from build123d import *

# Parameters (mm, degrees)
F1_R          = 28.006963647
F2_DEPTH      = 100
F0_R          = 228.6
F3_DEPTH      = 50
F4_R          = 7.5
F5_DEPTH      = 28.006963647
F5_DEPTH_BACK = 28.006963647


with BuildPart() as f2:
    # F1 (on Front) → F2 (new body)
    with BuildSketch(Plane.XZ):
        Circle(F1_R)
    extrude(amount=F2_DEPTH)

    # F0 (on Front) → F3 (join)
    with BuildSketch(Plane.XZ):
        Circle(F0_R)
    extrude(amount=-F3_DEPTH)

    # F4 (on Top) → F5 (cut, two sides)
    with BuildSketch(Plane.XY) as f5_sk:
        with Locations((0, -45)):
            Circle(F4_R)
    extrude(amount=-F5_DEPTH, mode=Mode.SUBTRACT)
    extrude(f5_sk.sketch, amount=F5_DEPTH_BACK, mode=Mode.SUBTRACT)


solid = f2.part
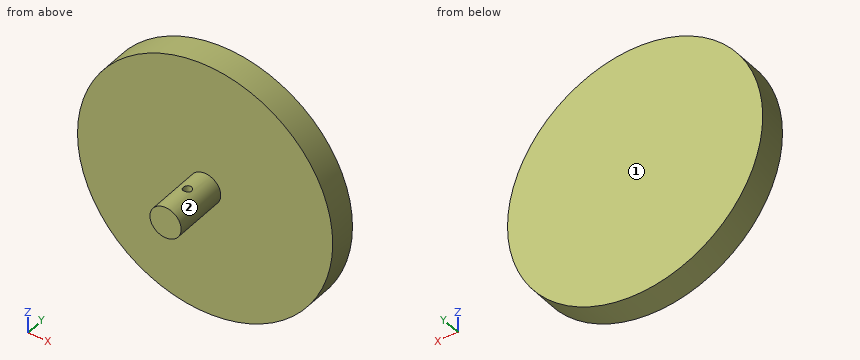
Geometry: final body of the model. Coordinates: model frame, mm. Face numbers are marked on the shaded views. A direction names the side the tool comes from. Round coordinates to 2 decimals unless told otherwise and drop trailing zeros. Loops run counter-clockwise (first coordinate to the right, second up) from the corner with the lowest first, then second, coordinate; pieces in that order, holes last. Notation, with made-up numbers: M 1,-22.5 L 13,-22.5 A25 cw 13,10.5 Z; hole C 5.5,13 d11. An arc over 180 degrees is marked long. Put each result on its own line as item: value. Start each with the question number.
(1) Section query A-A (z = 0). Return loops of the section in (x, y).
(2) Section query B-B (x = 0). Return loops of the section in (y, z).
(3) Section query D-D (y = -18). Return loops of the section in (x, z), then the cut area to 3 significant figures.
(4) Material intervals for line 1 along Y through (x, z) = (0, 0); line 2 along Y through (x, z) = (-159.5, 16); line 3 along X through (y, z) = (-45, 3), sorted ascending. Write a range as [from, to].
(5) Set-up query: the marked faces 1 and 2. Return all of +Z, -Z, +X, -X, +Y, -Y with unobstructed straight access to the full face (end or side cutting, diameter ignored); none if empty.
(6) Section query C-C (y = -45). Return loops of the section in (x, z).
(7) Contact query for flat-ended pins moving along their axis: pin 1 Ø10 at (y, z) = (-38, -16.5) entering from -X; pin 2 Ø24 at (x, y) = (0, -45) entering from +Z; pin 3 Ø5 at (x, y) = (-15.5, -67.5) entering from +Z; pin 4 Ø12 at (x, y) = (136.5, -10) entering from -Z. Output: stop coordinate, or through.
Findings below:
1. outline: M -228.6,0 L -28.01,0 L -28.01,-100 L 28.01,-100 L 28.01,0 L 228.6,0 L 228.6,50 L -228.6,50 Z; hole C 0,-45 d15
2. outline: M -100,-28.01 L -52.5,-28.01 L -52.5,28.01 L -100,28.01 Z; M -37.5,-28.01 L 0,-28.01 L 0,-228.6 L 50,-228.6 L 50,228.6 L 0,228.6 L 0,28.01 L -37.5,28.01 Z
3. outline: C 0,0 d56.01
3. area: 2,460 mm2
4. line 1: y = [-100, -52.5], [-37.5, 50]
4. line 2: y = [0, 50]
4. line 3: x = [-27.85, -7.5], [7.5, 27.85]
5. face 1: +Z, -Z, +X, -X, +Y
5. face 2: -Y
6. outline: M -7.5,-26.98 L -7.5,26.98 A28.01 ccw Z; M 7.5,-26.98 A28.01 ccw 7.5,26.98 Z
7. pin 1: stops at x = -25.54
7. pin 2: stops at z = 28.01
7. pin 3: stops at z = 24.81
7. pin 4: passes through
